Read the model definition and answer for the solid it produces. Units are mm, in the model's axes. Coordinates: 2 decimals unless noted, no trailing zeros. Loops run counter-clockwise (first coordinate to the right, second up) from the corner with the lowest first, then second, coordinate; pieces in that order, holes last.
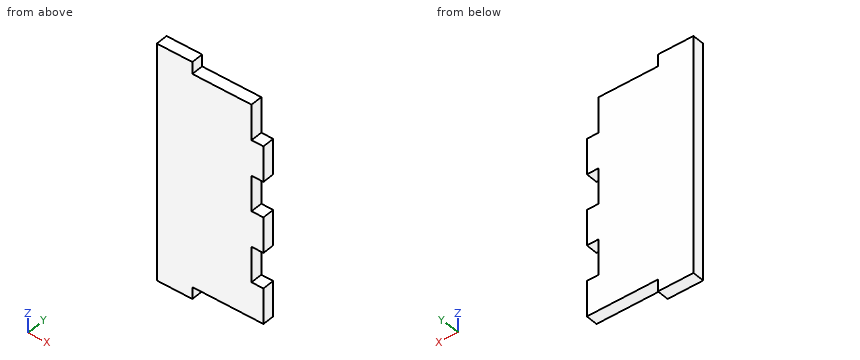
Autodesk Inventor part; units mm, degrees
ref_plane "YZ Plane" through (0, 0, 0) normal (1, 0, 0) x (0, 1, 0)
ref_plane "XZ Plane" through (0, 0, 0) normal (0, 1, 0) x (-1, 0, 0)
ref_plane "XY Plane" through (0, 0, 0) normal (0, 0, 1) x (1, 0, 0)
sketch "Sketch1" plane through (0, 0, 0) normal (0, 1, 0) x (-1, 0, 0)
  line L0 (0, 0) -> (60, 0)
  line L1 (60, 0) -> (60, -133.4)
  line L2 (60, -133.4) -> (0, -133.4)
  line L3 (0, -133.4) -> (0, 0)
  dimension "d0" = 133.4
  dimension "d1" = 60
extrude "Extrusion1" add sketch "Sketch1" along normal blind 6.7
sketch "Sketch2" plane through (0, 6.7, 0) normal (0, 1, 0) x (1, 0, 0)
  line L0 (0, 0) -> (0, 6.7)
  line L1 (0, 0) -> (0, 133.4)
  line L2 (0, 6.7) -> (-6.7, 6.7)
  line L3 (-6.7, 6.7) -> (-6.7, 26.7)
  line L4 (-6.7, 26.7) -> (0, 26.7)
  line L5 (0, 26.7) -> (0, 6.7)
  dimension "d4" = 6.7
  dimension "d5" = 6.7
  dimension "d6" = 20
extrude "Extrusion2" cut sketch "Sketch2" against normal blind 6.7
pattern_linear "Rectangular Pattern1" count 3 spacing 40 along (0, 0, -1) of "Extrusion2"
sketch "Sketch3" plane through (0, 6.7, 0) normal (0, 1, 0) x (1, 0, 0)
  line L0 (0, 0) -> (-60, 0)
  line L1 (-60, 0) -> (-40, 0)
  line L2 (-40, 0) -> (-20, 0)
  line L3 (0, 6.7) -> (0, 0)
  line L4 (-40, 0) -> (0, 0)
  line L5 (0, 0) -> (0, 6.7)
  line L6 (0, 6.7) -> (-40, 6.7)
  line L7 (-40, 6.7) -> (-40, 0)
  line L8 (-60, 133.4) -> (-40, 133.4)
  line L9 (-60, 133.4) -> (0, 133.4)
  line L10 (0, 133.4) -> (0, 106.7)
  line L11 (-40, 133.4) -> (0, 133.4)
  line L12 (0, 133.4) -> (0, 126.7)
  line L13 (0, 126.7) -> (-40, 126.7)
  line L14 (-40, 126.7) -> (-40, 133.4)
  dimension "d12" = 20
  dimension "d15" = 20
  dimension "d16" = 6.7
extrude "Extrusion3" cut sketch "Sketch3" against normal blind 6.7
properties part number "b_base_support 3"
Item 1: A cutting plane is placed at C-C on x = -36. Determine the outline of the cut face in (y, z).
Numbers:
outline: (0, -126.7) - (6.7, -126.7) - (6.7, -6.7) - (0, -6.7) - close
Item 2: A cutting plane is placed at B-B on z = -19.5. Determine the outline of the cut face in (x, y).
Numbers:
outline: (-60, 0) - (-6.7, 0) - (-6.7, 6.7) - (-60, 6.7) - close
Item 3: Find the intervals of material crossed by line 1 along Z through (x, y) = (-4.5, 4); line 2 along Z through (x, y) = (-14, 2.75); line 3 along X through (y, z) = (4.5, -50), in increasing order.
Numbers:
line 1: z = -126.7 to -106.7, -86.7 to -66.7, -46.7 to -26.7
line 2: z = -126.7 to -6.7
line 3: x = -60 to -6.7
Item 4: A cutting plane is placed at A-A on y = 1.25. Determine the outline of the cut face in (x, z), then the cut area to 3 significant figures.
Numbers:
outline: (-60, -133.4) - (-40, -133.4) - (-40, -126.7) - (0, -126.7) - (0, -106.7) - (-6.7, -106.7) - (-6.7, -86.7) - (0, -86.7) - (0, -66.7) - (-6.7, -66.7) - (-6.7, -46.7) - (0, -46.7) - (0, -26.7) - (-6.7, -26.7) - (-6.7, -6.7) - (-40, -6.7) - (-40, 0) - (-60, 0) - close
area: 7,070 mm2
Item 5: Given pin 1 (3.5 mm diameter, centred on x = -3.5, y = 4, fed in from +Z); pin 2 (4 mm diameter, centred on x = -9, y = 1, fed in from +Z); pin 3 (3.5 mm diameter, centred on y = 2, z = -3, fed in from +X), each flat-ended and moving along its own axis, determine where each tip first touches the part or whether it passes through.
Numbers:
pin 1: stops at z = -26.7
pin 2: stops at z = -6.7
pin 3: stops at x = -40
